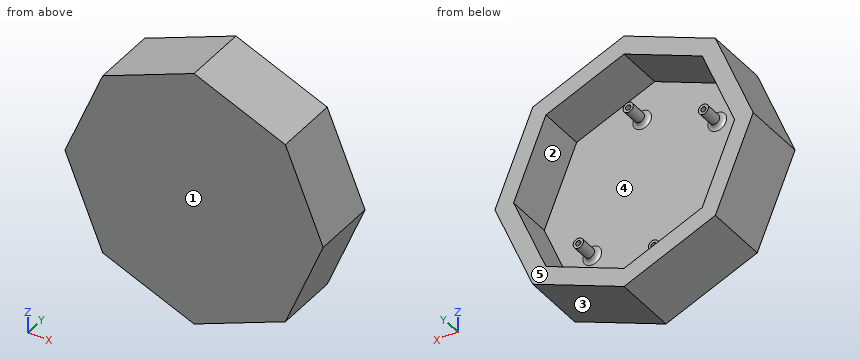
from build123d import *

# Parameters (mm, degrees)
BOSS_EXTRUDE1_DEPTH             = 38.1
SHELL1_T                        = -10.16
SKETCH5_R                       = 3.000653817
BOSS_EXTRUDE2_DEPTH             = 12.7
FILLET2_R                       = 2.54
TAP_DRILL_FOR_4_HELICOIL2_D     = 3.048
TAP_DRILL_FOR_4_HELICOIL2_DEPTH = 8.89
TAP_DRILL_FOR_4_HELICOIL2_TIP   = 0.915711583


with BuildPart() as part:
    # Sketch1 → Boss-Extrude1 (new body)
    with BuildSketch(Plane(origin=(0, 0, 0), x_dir=(1, 0, 0), z_dir=(0, 1, 0))):
        Polygon((76.2, 0), (53.881536726, 53.881536726), (0, 76.2), (-53.881536726, 53.881536726), (-76.2, 0), (-53.881536726, -53.881536726), (0, -76.2), (53.881536726, -53.881536726), align=None)
    extrude(amount=BOSS_EXTRUDE1_DEPTH)

    # Shell1
    shell1_openings = [part.faces().sort_by_distance(p)[0] for p in [
        (0, 38.1, 0),
    ]]
    offset(amount=SHELL1_T, openings=shell1_openings, kind=Kind.INTERSECTION)

    # Sketch5 → Boss-Extrude2 (add)
    with BuildSketch(Plane(origin=(0, 10.16, 0), x_dir=(1, 0, 0), z_dir=(0, 1, 0))):
        with Locations(Location((-7.439796634, 44.753764378, 0), (0, 0, 270))):
            Circle(SKETCH5_R)
        with Locations(Location((36.906420926, 26.384959625, 0), (0, 0, 90))):
            Circle(SKETCH5_R)
        with Locations(Location((7.439796634, -44.753764378, 0), (0, 0, 270))):
            Circle(SKETCH5_R)
        with Locations(Location((-36.906420926, -26.384959625, 0), (0, 0, 90))):
            Circle(SKETCH5_R)
    extrude(amount=BOSS_EXTRUDE2_DEPTH)

    # Fillet2
    fillet2_edges = [part.edges().sort_by_distance(p)[0] for p in [
        (-7.439796634, 10.16, -47.754418196),
        (36.906420926, 10.16, -23.384305808),
        (7.439796634, 10.16, 41.753110561),
        (-36.906420926, 10.16, 29.385613442),
    ]]
    fillet(fillet2_edges, radius=FILLET2_R)

    # Tap Drill for #4 Helicoil2
    with Locations(Plane(origin=(0, 22.86, 0), x_dir=(1, 0, 0), z_dir=(0, 1, 0))):
        with Locations((-7.439796634, 44.753764378), (36.906420926, 26.384959625), (7.439796634, -44.753764378), (-36.906420926, -26.384959625)):
            Hole(TAP_DRILL_FOR_4_HELICOIL2_D / 2, depth=TAP_DRILL_FOR_4_HELICOIL2_DEPTH)
            with Locations((0, 0, -(TAP_DRILL_FOR_4_HELICOIL2_DEPTH + TAP_DRILL_FOR_4_HELICOIL2_TIP / 2))):  # 118° drill point
                Cone(0, TAP_DRILL_FOR_4_HELICOIL2_D / 2, TAP_DRILL_FOR_4_HELICOIL2_TIP, mode=Mode.SUBTRACT)


solid = part.part
The listing builds one solid part. Answer for the finished solid, in the listing's coordinates (mm). Face numbers are marked on the shaded views. A direction names the side the tool comes from. Give positions to 0.01 mm unless a question says otherwise; leave off trailing zeros. Write each loop counter-clockwise with the first axis right and the second up, starting at its lowest first coordinate (ties: lowest second). Pieces come first, ordered by that corner, then holes.
Item 1: Determine the mould class of the marked faces 3, 4 and 5 for opening direction Z: released by +Z, released by -Z, zero draft, split by the parting line, or undercut.
Item 2: Section A-A, the plane y = 19 is taken. Count the separate pieces of the cut face and the enclosed holes in it, plus the area to 3 significant figures.
Item 3: Flat-ended cylindrical pins translate along their axes: P1, Ø8, axis at y = 29.5, z = -23.5, coming from the -X side; P2, Ø5, axis at x = -37.5, z = 27.5, coming from the +Y side; P3, Ø10, axis at x = 3.5, y = 28.5, coming from the +Z side; P4, Ø6, axis at x = -48.5, z = 25.5, coming from the -Y side. Find the tip coordinate at first contact, or state that the pin passes through.
Item 4: Section B-B, the plane y = 35 is taken. Write down the section's boundary in (x, z), plus the area to 3 significant figures.
Item 5: Section C-C, the plane z = -17 is taken. Write down the section's boundary in (x, y), plus the area to 3 significant figures.
Item 6: Section D-D, the plane x = -49.5 is taken. Write down the section's boundary in (y, z).
Item 7: Which of the six approach directions +Z, -Z, +X, -X, +Y, -Y give full straight-line access (tool end or side, diameter ignored) to the marked faces 1 and 2?
Item 8: Find the intervals of material crossed by line 1 along Y through (x, z) = (31.5, -10); line 2 along X through (y, z) = (23.5, 38); line 3 along Z through (x, y) = (-41, 31), in increasing order.
Completed:
1. face 3: released by -Z
1. face 4: undercut
1. face 5: zero draft
2. separate pieces: 5
2. enclosed holes: 5
2. area: 4,480 mm2
3. P1: stops at x = -68.12
3. P2: stops at y = 22.86
3. P3: stops at z = 76.2
3. P4: stops at y = 0
4. outline: (-76.2, 0) - (-53.88, -53.88) - (0, -76.2) - (53.88, -53.88) - (76.2, 0) - (53.88, 53.88) - (0, 76.2) - (-53.88, 53.88) - close; hole (-65.2, 0) - (-46.11, -46.11) - (0, -65.2) - (46.11, -46.11) - (65.2, 0) - (46.11, 46.11) - (0, 65.2) - (-46.11, 46.11) - close
4. area: 4,400 mm2
5. outline: (-69.16, 0) - (69.16, 0) - (69.16, 38.1) - (58.16, 38.1) - (58.16, 10.16) - (-58.16, 10.16) - (-58.16, 38.1) - (-69.16, 38.1) - close
5. area: 2,020 mm2
6. outline: (0, -55.7) - (38.1, -55.7) - (38.1, -37.91) - (10.16, -37.91) - (10.16, 37.91) - (38.1, 37.91) - (38.1, 55.7) - (0, 55.7) - close
7. face 1: +Z, -Z, +X, -X, -Y
7. face 2: +Y
8. line 1: y = 0 to 10.16
8. line 2: x = -60.46 to -49.46, 49.46 to 60.46
8. line 3: z = -59.22 to -48.22, 48.22 to 59.22
